from build123d import *

# Parameters (mm, degrees)
BOSS_EXTRUDE1_DEPTH   = 25.4
M10_CLEARANCE_HOLE1_D = 11
M5_CLEARANCE_HOLE2_D  = 5.5


with BuildPart() as part:
    # Sketch1 → Boss-Extrude1 (new body)
    with BuildSketch(Plane.XY):
        Polygon((0, 0), (15.875, 0), (15.875, 3.175), (3.175, 3.175), (3.175, 28.575), (0, 28.575), align=None)
    extrude(amount=BOSS_EXTRUDE1_DEPTH)

    # M10 Clearance Hole1 (through all)
    with Locations(Plane(origin=(3.175, 0, 0), x_dir=(0, 0, -1), z_dir=(1, 0, 0))):
        with Locations((-12.7, 19.05)):
            Hole(M10_CLEARANCE_HOLE1_D / 2)

    # M5 Clearance Hole2 (through all)
    with Locations(Plane(origin=(0, 3.175, 0), x_dir=(1, 0, 0), z_dir=(0, 1, 0))):
        with Locations((6.35, -19.05), (6.35, -6.35)):
            Hole(M5_CLEARANCE_HOLE2_D / 2)


solid = part.part
Design review of the part built by this model. Coordinates are the model's own, in mm. A direction names the side the tool comes from. Coordinates: 2 decimals unless noted, no trailing zeros. Loops run counter-clockwise (first coordinate to the right, second up) from the corner with the lowest first, then second, coordinate; pieces in that order, holes last. Notation, with made-up numbers: (42.5, 59.25) - (51.5, 59.25) arc R6 cw to (51.5, 67.25) - close; hole circle Ø1 at (19.5, 10.25). An arc over 180 degrees is marked (long way). Use CSV: the item, a comma, the result in double quotes. Start each with the question number.
1. To check wall thickness, follow probe 1 along Z at (x, y) = (6.35, 1.45); probe 2 along Y at (x, z) = (2.05, 12.7) (3 decimals); probe 3 along X at (y, z) = (2.4, 19.05) (3 decimals). State the ranges of each line that lie inside material, in increasing order.
2. Add section C-C on x = 6.35. Give the boundary of the cut face in (y, z) (3 decimals).
3. Add section B-B on y = 20.5. Give the boundary of the cut face in (x, z) (3 decimals).
4. Mouldability with a two-part tool opening along Z and no side actions: class faces 3 (the flat face through (0, 11, 13)), 4 (the flat face through (3, 12, 25.4)), 5 (the cylindrical face through (6.708, 1.565, 16.323)) as released by +Z, released by -Z, zero draft, split by the parting line, or undercut.
5. Add section D-D on y = 2.5. Give the boundary of the cut face in (x, z) (3 decimals), plus the area to 3 significant figures.
6. Add section A-A on z = 19.05. Give the boundary of the cut face in (x, y) (3 decimals).
7. For faces 1 (the flat face through (8, 0, 13)), 2 (the flat face through (3.175, 13, 13)), list the 3-axis set-ups (+Z, -Z, +X, -X, +Y, -Y) from which the entire face can be reached by the end or side of a thin tool; tool diameter is ignored.
8. Clearance check with flat-ended pins moving along their axes: pin 1 (8 mm diameter, centred on x = 3, z = 14, fed in from -Y); pin 2 (4.5 mm diameter, centred on x = 6.35, z = 19.05, fed in from +Y); pin 3 (12.5 mm diameter, centred on y = 10, z = 14.5, fed in from +X) (3 decimals); pin 4 (8 mm diameter, centred on x = 13, z = 17, fed in from +Y) (3 decimals). State where each tip first meets the part, or that it passes through.
Resolved:
1,probe 1,"0 to 3.6, 9.1 to 16.3, 21.8 to 25.4"
1,probe 2,"0 to 13.55, 24.55 to 28.575"
1,probe 3,"0 to 3.6, 9.1 to 15.875"
2,outline,"(0, 0) - (3.175, 0) - (3.175, 3.6) - (0, 3.6) - close; (0, 9.1) - (3.175, 9.1) - (3.175, 16.3) - (0, 16.3) - close; (0, 21.8) - (3.175, 21.8) - (3.175, 25.4) - (0, 25.4) - close"
3,outline,"(0, 0) - (3.175, 0) - (3.175, 7.395) - (0, 7.395) - close; (0, 18.005) - (3.175, 18.005) - (3.175, 25.4) - (0, 25.4) - close"
4,face 3,"zero draft"
4,face 4,"released by +Z"
4,face 5,"undercut"
5,outline,"(0, 0) - (15.875, 0) - (15.875, 25.4) - (0, 25.4) - close; hole circle Ø5.5 at (6.35, 6.35); hole circle Ø5.5 at (6.35, 19.05)"
5,area,"356 mm2"
6,outline,"(0, 0) - (3.6, 0) - (3.6, 3.175) - (3.175, 3.175) - (3.175, 28.575) - (0, 28.575) - close; (9.1, 0) - (15.875, 0) - (15.875, 3.175) - (9.1, 3.175) - close"
7,face 1,"+Z, -Z, +X, -X, -Y"
7,face 2,"+Z, -Z, +X, +Y"
8,pin 1,"y = 0"
8,pin 2,"through"
8,pin 3,"x = 3.175"
8,pin 4,"y = 3.175"
